Design review of the part built by this model. Coordinates are the model's own, in mm. Face numbers are marked on the shaded views. A direction names the side the tool comes from. Round coordinates to 2 decimals unless told otherwise and drop trailing zeros. Loops run counter-clockwise (first coordinate to the right, second up) from the corner with the lowest first, then second, coordinate; pieces in that order, holes last. Notation, with made-up numbers: (39, -12) -> (97, -12) arc R20 cw to (97, 2) -> close; hole circle Ø4 at (-15, 60). An arc over 180 degrees is marked (long way). Use a Markdown table: item, result. Add a question column.
from build123d import *


with BuildPart() as part:
    # Esquisse1 → Révolution1 (revolve)
    with BuildSketch(Plane(origin=(0, 0, 0), x_dir=(0, 0, -1), z_dir=(1, 0, 0))):
        with BuildLine():
            Line((97.44, 0), (97.44, 8.03))
            ThreePointArc((97.44, 8.03), (96.854213562, 9.444213562), (95.44, 10.03))
            Line((95.44, 10.03), (91.34, 10.03))
            Line((91.34, 10.03), (91.34, 5.53))
            Line((91.34, 5.53), (43, 5.53))
            Line((43, 5.53), (40.5, 4))
            Line((40.5, 4), (0, 4))
            Line((0, 4), (0, 0))
            Line((0, 0), (97.44, 0))
        make_face()
    revolve(axis=Axis((0, 0, 0), (0, 0, -1)))


solid = part.part
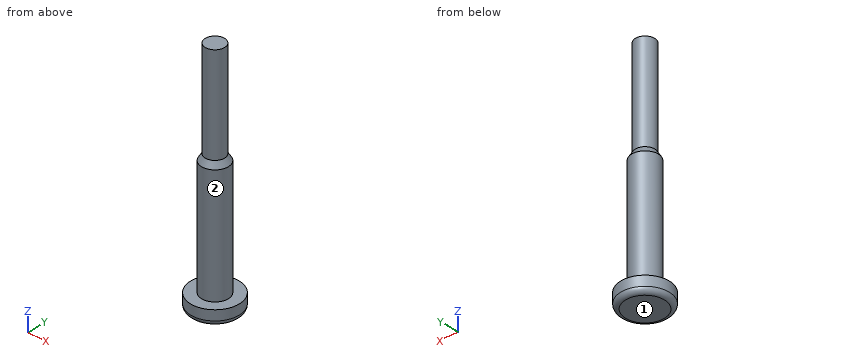
1. Consider section C-C on z = -65. State the section outline as (x, y) points.
2. Consider section A-A on y = 0. State the section outline as (x, z) points.
3. Insertion check: P1, Ø12, axis at y = -7, z = -11, coming from the -X side; P2, Ø1, axis at x = -5, z = -34.5, coming from the +Y side; P3, Ø6, axis at x = -7, y = 1, coming from the +Z side; P4, Ø1, axis at y = 3.5, z = -65.5, coming from the +X side. Each pin has a flat end and moves straight along its axis. Give the tip position at first contact, or say it passes through.
4. To check wall thickness, follow probe 1 along Y at (x, z) = (0.25, -33.5); probe 2 along Z at (x, y) = (7, 4); probe 3 along X at (y, z) = (2, -70). State the ranges of each line that lie inside material, in increasing order. Write a range as from..to.
5. For the marked faces 1 and 2, list the 3-axis set-ups (+Z, -Z, +X, -X, +Y, -Y) from which the entire face can be reached by the end or side of a thin tool; tool diameter is ignored.
6. Consider section D-D on z = -14. State the section outline as (x, y) points, plus the area to 3 significant figures.
Verdict:
| question | item | result |
|---|---|---|
| 1 | outline | circle Ø11.06 at (0, 0) |
| 2 | outline | (-10.03, -95.44) arc R2 ccw to (-8.03, -97.44) -> (8.03, -97.44) arc R2 ccw to (10.03, -95.44) -> (10.03, -91.34) -> (5.53, -91.34) -> (5.53, -43) -> (4, -40.5) -> (4, 0) -> (-4, 0) -> (-4, -40.5) -> (-5.53, -43) -> (-5.53, -91.34) -> (-10.03, -91.34) -> close |
| 3 | P1 | stops at x = -3.87 |
| 3 | P2 | passes through |
| 3 | P3 | stops at z = -40.62 |
| 3 | P4 | stops at x = 4.65 |
| 4 | probe 1 | y = -3.99..3.99 |
| 4 | probe 2 | z = -97.44..-91.34 |
| 4 | probe 3 | x = -5.16..5.16 |
| 5 | face 1 | -Z, +X, -X, +Y, -Y |
| 5 | face 2 | +Z |
| 6 | outline | circle Ø8 at (0, 0) |
| 6 | area | 50.3 mm² |
